```python
from build123d import *

# Parameters (mm, degrees)
SKETCH1_R           = 1.778
BOSS_EXTRUDE1_DEPTH = 2.54
FILLET1_R           = 2.54


with BuildPart() as part:
    # Sketch1 → Boss-Extrude1 (new, symmetric)
    with BuildSketch(Plane.XY):
        with BuildLine():
            ThreePointArc((23.096897519, 13.335), (18.163878776, 19.528502447), (11.629866574, 24.000731311))
            add(Edge.make_bspline(
                [(12.942718979, 26.367649013), (12.489890773, 26.524403161), (10.214611, 26.823602727), (8.514999239, 25.805149786), (11.629866574, 24.000731311)],
                knots=[0.119187678, 0.119187678, 0.119187678, 0.119187678, 0.354139338, 1, 1, 1, 1], degree=3))
            ThreePointArc((12.942718979, 26.367649013), (14.594299506, 26.395047723), (14.579783558, 28.046791715))
            ThreePointArc((14.579783558, 28.046791715), (0, 32.207688222), (-14.579783558, 28.046791715))
            ThreePointArc((-14.579783558, 28.046791715), (-14.594299506, 26.395047723), (-12.942718979, 26.367649013))
            add(Edge.make_bspline(
                [(-12.942718979, 26.367649013), (-12.489890773, 26.524403161), (-10.214611, 26.823602727), (-8.514999239, 25.805149786), (-11.629866574, 24.000731311)],
                knots=[0.119187678, 0.119187678, 0.119187678, 0.119187678, 0.354139338, 1, 1, 1, 1], degree=3))
            ThreePointArc((-11.629866574, 24.000731311), (-18.163878776, 19.528502447), (-23.096897519, 13.335))
            ThreePointArc((-23.096897519, 13.335), (-23.564242622, 12.49061126), (-24.000731311, 11.629866574))
            add(Edge.make_bspline(
                [(-26.367649013, 12.942718979), (-26.524403161, 12.489890773), (-26.823602727, 10.214611), (-25.805149786, 8.514999239), (-24.000731311, 11.629866574)],
                knots=[0.119187678, 0.119187678, 0.119187678, 0.119187678, 0.354139338, 1, 1, 1, 1], degree=3))
            ThreePointArc((-26.367649013, 12.942718979), (-26.395047723, 14.594299506), (-28.046791715, 14.579783558))
            ThreePointArc((-28.046791715, 14.579783558), (-32.207688222, 0), (-28.046791715, -14.579783558))
            ThreePointArc((-28.046791715, -14.579783558), (-26.395047723, -14.594299506), (-26.367649013, -12.942718979))
            add(Edge.make_bspline(
                [(-26.367649013, -12.942718979), (-26.524403161, -12.489890773), (-26.823602727, -10.214611), (-25.805149786, -8.514999239), (-24.000731311, -11.629866574)],
                knots=[0.119187678, 0.119187678, 0.119187678, 0.119187678, 0.354139338, 1, 1, 1, 1], degree=3))
            ThreePointArc((-24.000731311, -11.629866574), (-18.858537854, -18.858537854), (-11.629866574, -24.000731311))
            add(Edge.make_bspline(
                [(-12.942718979, -26.367649013), (-12.489890773, -26.524403161), (-10.214611, -26.823602727), (-8.514999239, -25.805149786), (-11.629866574, -24.000731311)],
                knots=[0.119187678, 0.119187678, 0.119187678, 0.119187678, 0.354139338, 1, 1, 1, 1], degree=3))
            ThreePointArc((-12.942718979, -26.367649013), (-14.594299506, -26.395047723), (-14.579783558, -28.046791715))
            ThreePointArc((-14.579783558, -28.046791715), (0, -32.207688222), (14.579783558, -28.046791715))
            ThreePointArc((14.579783558, -28.046791715), (14.594299506, -26.395047723), (12.942718979, -26.367649013))
            add(Edge.make_bspline(
                [(12.942718979, -26.367649013), (12.489890773, -26.524403161), (10.214611, -26.823602727), (8.514999239, -25.805149786), (11.629866574, -24.000731311)],
                knots=[0.119187678, 0.119187678, 0.119187678, 0.119187678, 0.354139338, 1, 1, 1, 1], degree=3))
            ThreePointArc((11.629866574, -24.000731311), (18.858537854, -18.858537854), (24.000731311, -11.629866574))
            add(Edge.make_bspline(
                [(26.367649013, -12.942718979), (26.524403161, -12.489890773), (26.823602727, -10.214611), (25.805149786, -8.514999239), (24.000731311, -11.629866574)],
                knots=[0.119187678, 0.119187678, 0.119187678, 0.119187678, 0.354139338, 1, 1, 1, 1], degree=3))
            ThreePointArc((26.367649013, -12.942718979), (26.395047723, -14.594299506), (28.046791715, -14.579783558))
            ThreePointArc((28.046791715, -14.579783558), (32.207688222, 0), (28.046791715, 14.579783558))
            ThreePointArc((28.046791715, 14.579783558), (26.395047723, 14.594299506), (26.367649013, 12.942718979))
            add(Edge.make_bspline(
                [(26.367649013, 12.942718979), (26.524403161, 12.489890773), (26.823602727, 10.214611), (25.805149786, 8.514999239), (24.000731311, 11.629866574)],
                knots=[0.119187678, 0.119187678, 0.119187678, 0.119187678, 0.354139338, 1, 1, 1, 1], degree=3))
            ThreePointArc((24.000731311, 11.629866574), (23.564242622, 12.49061126), (23.096897519, 13.335))
        make_face()
        with Locations((0, 17.78)):
            Circle(SKETCH1_R, mode=Mode.SUBTRACT)
        with Locations((15.397931679, -8.89)):
            Circle(SKETCH1_R, mode=Mode.SUBTRACT)
        with Locations((-15.397931679, -8.89)):
            Circle(SKETCH1_R, mode=Mode.SUBTRACT)
        with BuildLine():
            Line((-4.28625, 20.274952091), (-4.28625, 22.454568821))
            ThreePointArc((-4.28625, 22.454568821), (-13.24349331, 18.633021359), (-19.797340731, 11.43))
            ThreePointArc((-19.797340731, 11.43), (-22.758416501, 2.152690962), (-21.58935203, -7.515283024))
            Line((-21.58935203, -7.515283024), (-17.877685951, -4.59493961))
            ThreePointArc((-17.877685951, -4.59493961), (-10.605148477, -7.614870918), (-15.415498572, -13.849477433))
            Line((-15.415498572, -13.849477433), (-17.30310203, -14.939285797))
            ThreePointArc((-17.30310203, -14.939285797), (-9.514923191, -20.78571232), (0, -22.86))
            ThreePointArc((0, -22.86), (9.514923191, -20.78571232), (17.30310203, -14.939285797))
            Line((17.30310203, -14.939285797), (12.918177407, -13.18506039))
            ThreePointArc((12.918177407, -13.18506039), (11.8972459, -5.376892533), (19.701748572, -6.425474659))
            Line((19.701748572, -6.425474659), (21.58935203, -7.515283024))
            ThreePointArc((21.58935203, -7.515283024), (22.758416501, 2.152690962), (19.797340731, 11.43))
            ThreePointArc((19.797340731, 11.43), (13.24349331, 18.633021359), (4.28625, 22.454568821))
            Line((4.28625, 22.454568821), (4.959508544, 17.78))
            ThreePointArc((4.959508544, 17.78), (-1.292097423, 12.991763451), (-4.28625, 20.274952091))
        make_face(mode=Mode.SUBTRACT)
    extrude(amount=BOSS_EXTRUDE1_DEPTH, both=True)

    # Fillet1
    # the kernel refuses this fillet: 2.54 mm, written as the material it adds along each edge
    with BuildSketch(Plane(origin=(21.58935203, -7.515283024, 0), x_dir=(-0.8660254037844372, 0.5000000000000026, 0), z_dir=(0, 0, -1)), Plane(origin=(-17.30310203, -14.939285797, 0), x_dir=(0.8660254037844382, 0.5000000000000008, 0), z_dir=(0, 0, -1)), Plane(origin=(-4.28625, 22.454568821, 0), x_dir=(0, -1, 0), z_dir=(0, 0, -1))) as fillet1_piece_1:
        with BuildLine():
            CenterArc((3.235105636, 2.310312353), FILLET1_R, 161.0565991, 84.38964425)
            Line((0.832672738, 3.134882647), (0.78462408, 3.151374053))
            ThreePointArc((0.78462408, 3.151374053), (0.311567983, 1.595269408), (-0.049899042, 0.009525))
            Line((-0.049899042, 0.009525), (0, -0.0508))
            ThreePointArc((0, -0.0508), (1.089808365, -0.0508), (2.158506952, -0.046206247))
            Line((2.158506952, -0.046206247), (2.17961673, 0))
        make_face()
    extrude(amount=2.54)
    with BuildSketch(Plane(origin=(17.30310203, -14.939285797, 0), x_dir=(-0.7195709341275718, -0.6944189447003685, 0), z_dir=(0, 0, -1)), Plane(origin=(4.28625, 22.454568821, 0), x_dir=(0.9611699140434871, -0.2759572364291899, 0), z_dir=(0, 0, -1)), Plane(origin=(-21.58935203, -7.515283024, 0), x_dir=(-0.24159897991591575, 0.9703761811295601, 0), z_dir=(0, 0, -1))) as fillet1_piece_2:
        with BuildLine():
            CenterArc((3.922629513, 2.529497521), FILLET1_R, 155.785220789, 119.426923656)
            Line((1.60611307, 3.571299597), (1.559782741, 3.592135639))
            Line((1.559782741, 3.592135639), (-0.046330329, 0.020836042))
            Line((-0.046330329, 0.020836042), (-0.004614858, -0.05058995))
            ThreePointArc((-0.004614858, -0.05058995), (2.076686213, -0.145322312), (4.157987284, -0.05058995))
            Line((4.157987284, -0.05058995), (4.153372426, 0))
        make_face()
    extrude(amount=2.54)
    with BuildSketch(Plane(origin=(-21.58935203, -7.515283024, 0), x_dir=(-0.24159897991591575, 0.9703761811295601, 0), z_dir=(0, 0, 1)), Plane(origin=(4.28625, 22.454568821, 0), x_dir=(0.9611699140434871, -0.2759572364291899, 0), z_dir=(0, 0, 1)), Plane(origin=(17.30310203, -14.939285797, 0), x_dir=(-0.7195709341275718, -0.6944189447003685, 0), z_dir=(0, 0, 1))) as fillet1_piece_3:
        with BuildLine():
            CenterArc((3.922629513, -2.529497521), FILLET1_R, 84.787855555, 119.426923656)
            Line((1.60611307, -3.571299597), (1.559782741, -3.592135639))
            Line((1.559782741, -3.592135639), (-0.046330329, -0.020836042))
            Line((-0.046330329, -0.020836042), (-0.004614858, 0.05058995))
            ThreePointArc((-0.004614858, 0.05058995), (2.076686213, 0.145322312), (4.157987284, 0.05058995))
            Line((4.157987284, 0.05058995), (4.153372426, 0))
        make_face()
    extrude(amount=2.54)
    with BuildSketch(Plane(origin=(-4.28625, 22.454568821, 0), x_dir=(0, -1, 0), z_dir=(0, 0, 1)), Plane(origin=(-17.30310203, -14.939285797, 0), x_dir=(0.8660254037844382, 0.5000000000000008, 0), z_dir=(0, 0, 1)), Plane(origin=(21.58935203, -7.515283024, 0), x_dir=(-0.8660254037844372, 0.5000000000000026, 0), z_dir=(0, 0, 1))) as fillet1_piece_4:
        with BuildLine():
            CenterArc((3.235105636, -2.310312353), FILLET1_R, 114.55375665, 84.38964425)
            Line((0.832672738, -3.134882647), (0.78462408, -3.151374053))
            ThreePointArc((0.78462408, -3.151374053), (0.311567983, -1.595269408), (-0.049899042, -0.009525))
            Line((-0.049899042, -0.009525), (0, 0.0508))
            ThreePointArc((0, 0.0508), (1.089808365, 0.0508), (2.158506952, 0.046206247))
            Line((2.158506952, 0.046206247), (2.17961673, 0))
        make_face()
    extrude(amount=2.54)


solid = part.part
```
Could you check a few things on this model? Use its own coordinates, in mm. A direction names the side the tool comes from. Coordinates: 2 decimals unless noted, no trailing zeros. Order: outer loops, then holes, each group sorted by start corner. A loop starts at its lowest first (then second) coordinate and runs counter-clockwise, first axis right, second up. Notation, with made-up numbers: M -9.5,33.25 L -4.5,33.25 A26 cw -4.5,48.25 Z; hole C 26,16 d3. An arc over 180 degrees is marked long. Use a Markdown table: item, result. Add a question column.
Q1. I want a section at C-C on y = -8.89. List the corners of the cut face in (x, z) for me.
Q2. I want a section at A-A on x = 0. List the corners of the cut face in (y, z) for me, then the cut area to 3 significant figures.
Q3. I want a section at D-D on z = -1.4. Give the number of separate pieces and of enclosed holes in the cut face, then the cut area to 3 significant figures.
Q4. Which directions (+Z, -Z, +X, -X, +Y, -Y) give clear straight access to the entire face, cutting with the end or side of a thin tool? Please do faces 1 (the cylindrical face through (20.128, 10.837, 0.036)), 2 (the cylindrical face through (-32.207, 0.215, 0.036)).
Q5. I'm going to push flat-ended pins straight in: pin 1 (2 mm diameter, centred on x = 15.4, y = -8.89, fed in from +Z); pin 2 (1 mm diameter, centred on y = 21.5, z = -1, fed in from +X); pin 3 (1 mm diameter, centred on x = 19, z = -1.5, fed in from -Y); pin 4 (1 mm diameter, centred on y = -2, z = 0.5, fed in from -X). Where does each tip first touch, or does it pass through?
Q6. If I drill on L1, parallel to Y at x = 13.5, z = -1.45; L2, parallel to Y at x = -4.5, z = 1.7; L3, parallel to Y at x = -14, z = -0.85, over which ranges is the centre line in solid material (lowest first)?
Q7. We'd pull the mould along X, two halves only. Please class faces 3 (the flat face through (2, 14, -2.54)), 4 (the cylindrical face through (-10.64, -7.49, 0.04)), 5 (the cylindrical face through (32.207, -0.215, 0.036)): pulls with the +X half, pulls with the -X half, needs draft (parallel to the pull), parting line crosses it, or undercut.
Q8. I want a section at B-B on y = -16. List the corners of the cut face in (x, z) for me, then the cut area to 3 significant figures.
Checked values:
| question | item | result |
|---|---|---|
| 1 | outline | M -30.74,-2.54 L -17.18,-2.54 L -17.18,2.54 L -30.74,2.54 Z; M -13.62,-2.54 L -10.44,-2.54 L -10.44,2.54 L -13.62,2.54 Z; M 10.44,-2.54 L 13.62,-2.54 L 13.62,2.54 L 10.44,2.54 Z; M 17.18,-2.54 L 30.74,-2.54 L 30.74,2.54 L 17.18,2.54 Z |
| 2 | outline | M -32.21,-2.54 L -22.86,-2.54 L -22.86,2.54 L -32.21,2.54 Z; M 12.82,-2.54 L 16,-2.54 L 16,2.54 L 12.82,2.54 Z; M 19.56,-2.54 L 32.21,-2.54 L 32.21,2.54 L 19.56,2.54 Z |
| 2 | area | 128 mm² |
| 3 | separate pieces | 1 |
| 3 | enclosed holes | 4 |
| 3 | area | 1,390 mm² |
| 4 | face 1 | +Z, -Z |
| 4 | face 2 | +Z, -Z, -X |
| 5 | pin 1 | through |
| 5 | pin 2 | x = 16.44 |
| 5 | pin 3 | y = -19.21 |
| 5 | pin 4 | x = -32.17 |
| 6 | L1 | -28.68 to -26.07, -23 to -18.45, -13.42 to -4.31, 18.45 to 23, 26.07 to 28.68 |
| 6 | L2 | -31.84 to -22.41, 15.7 to 19.86, 20.65 to 31.84 |
| 6 | L3 | -28.4 to -26.07, -22.7 to -18.07, -13.65 to -9.99, -7.79 to -4.13, 18.07 to 22.7, 26.07 to 28.4 |
| 7 | face 3 | needs draft |
| 7 | face 4 | undercut |
| 7 | face 5 | pulls with the +X half |
| 8 | outline | M -21.34,-2.54 L -15.79,-2.54 L -15.79,2.54 L -21.34,2.54 Z; M 15.26,-2.54 L 21.34,-2.54 L 21.34,2.54 L 15.26,2.54 Z |
| 8 | area | 59.0 mm² |
